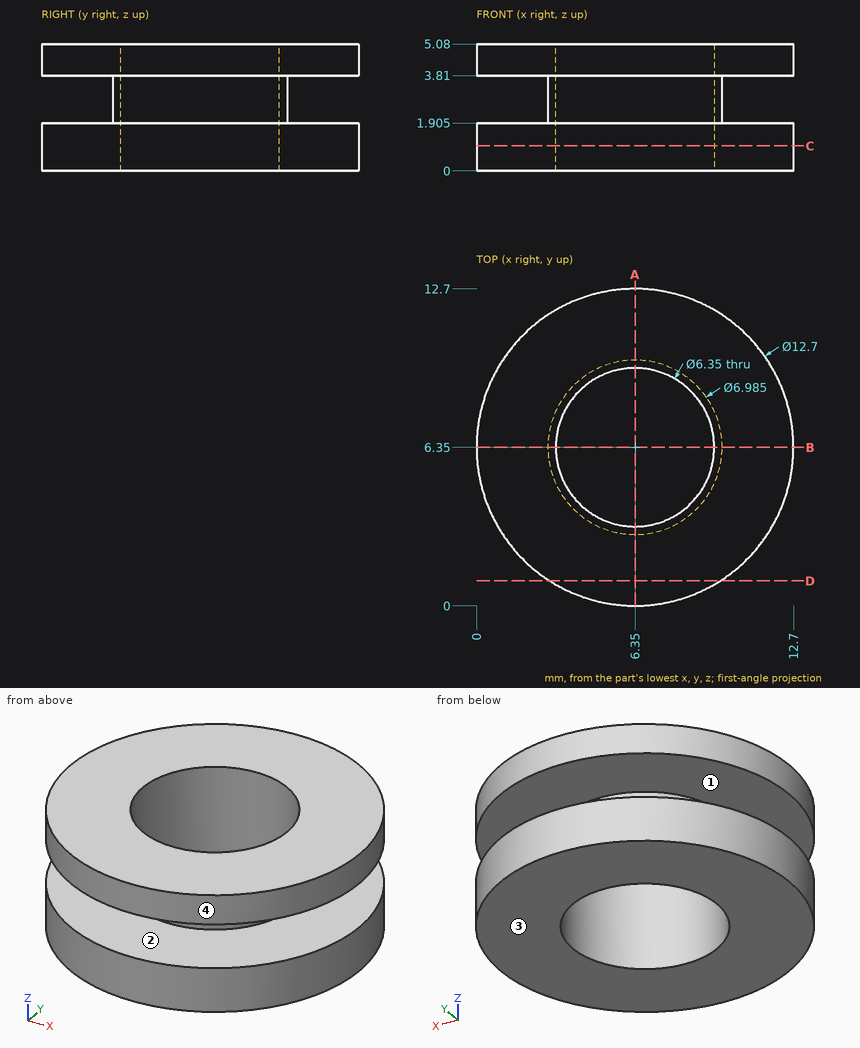
Source: three-view drawing plus pictorial views. Frame: mm from the lowest corner of the part. Give positions to 0.01 mm unless a question says otherwise; leave off trailing zeros. Order: outer loops, then holes, each group sorted by start corner. A loop starts at its lowest first (then second) coordinate and runs counter-clockwise, first axis right, second up. Notation, with made-up numbers: (72, -21) - (94, -21) arc R15 cw to (94, -16) - close; hole circle Ø9 at (-19.5, 54.5). An arc over 180 degrees is marked (long way). Put each result on its own line as item: value.
Item 1: Ray query, L1, parallel to Z at x = 2, y = 8 (3 decimals); L2, parallel to Y at x = 6.35, z = 2.1 (1 decimal); L3, parallel to Y at x = 6.35, z = 1.55 (3 decimals). Return the intervals inside material, ascending. Write a range as from..to.
Found:
L1: z = 0..1.905, 3.81..5.08
L2: y = 2.9..3.2, 9.5..9.8
L3: y = 0..3.175, 9.525..12.7
Item 2: Section query C-C, the plane z = 1. Return loops of the section in (x, y) (3 decimals).
Found:
outline: circle Ø12.7 at (6.35, 6.35); hole circle Ø6.35 at (6.35, 6.35)
Item 3: Draft query along Z for the marked faces 1, 2, 3 and 4. Return one class per face: +Z half, -Z half, draft (parallel to the pull), parting line (faces both ways), or undercut.
Found:
face 1: undercut
face 2: undercut
face 3: -Z half
face 4: draft
Item 4: Section query D-D, the plane y = 1. Return loops of the section in (x, z) (3 decimals).
Found:
outline: (2.929, 0) - (9.771, 0) - (9.771, 1.905) - (2.929, 1.905) - close; (2.929, 3.81) - (9.771, 3.81) - (9.771, 5.08) - (2.929, 5.08) - close
Item 5: Section query A-A, the plane x = 6.35. Return loops of the section in (y, z) (1 decimal).
Found:
outline: (0, 0) - (3.2, 0) - (3.2, 5.1) - (0, 5.1) - (0, 3.8) - (2.9, 3.8) - (2.9, 1.9) - (0, 1.9) - close; (9.5, 0) - (12.7, 0) - (12.7, 1.9) - (9.8, 1.9) - (9.8, 3.8) - (12.7, 3.8) - (12.7, 5.1) - (9.5, 5.1) - close
Item 6: Contact query for a flat-ended pin moving along its axis: pin 1 (2 mm diameter, centred on x = 3.5, z = 3.5, fed in from -Y). Output: stop coordinate, or through.
Found:
pin 1: stops at y = 0.29
